```python
from build123d import *

# Parameters (mm, degrees)
SKETCH1_R                           = 1.5
BOSS_EXTRUDE1_DEPTH                 = 42
SKETCH2_R                           = 2.75
BOSS_EXTRUDE2_DEPTH                 = 2.2
ESCALA1_SCALE                       = 1.5
ESCALA2_SCALE                       = 1.5
CROQUIS1_R                          = 3.4
SALIENTE_EXTRUIR1_DEPTH             = 10
SALIENTE_EXTRUIR1_DIRECTION_2_REACH = 96.904


with BuildPart() as part:
    # Sketch1 → Boss-Extrude1 (new body)
    with BuildSketch(Plane.XY):
        with Locations(Location((0, 0, 0), (0, 0, 180))):
            Circle(SKETCH1_R)
    extrude(amount=BOSS_EXTRUDE1_DEPTH)

    # Sketch2 → Boss-Extrude2 (add)
    with BuildSketch(Plane(origin=(0, 0, 0), x_dir=(-1, 0, 0), z_dir=(0, 0, -1))):
        Circle(SKETCH2_R)
    extrude(amount=-BOSS_EXTRUDE2_DEPTH)


with BuildPart() as part_1:
    # Escala1: scaled about (0, 0, 0)
    add(part.part.scale(ESCALA1_SCALE))


with BuildPart() as part_2:
    # Escala2: scaled about (0, 0, 0)
    add(part_1.part.scale(ESCALA2_SCALE))

    # Croquis1 → Saliente-Extruir1 (add)
    with BuildSketch(Plane.XY.offset(94.5)):
        Circle(CROQUIS1_R)
    extrude(amount=SALIENTE_EXTRUIR1_DEPTH)

    # Croquis1 → Saliente-Extruir1 direction 2 (add, up to next)
    with BuildSketch(Plane.XY.offset(94.5), mode=Mode.PRIVATE) as saliente_extruir1_direction_2_sk1:
        Circle(CROQUIS1_R)
    saliente_extruir1_direction_2_tool1 = extrude(saliente_extruir1_direction_2_sk1.sketch, amount=-SALIENTE_EXTRUIR1_DIRECTION_2_REACH, mode=Mode.PRIVATE) - part_2.part
    add(saliente_extruir1_direction_2_tool1.solids().sort_by_distance((0, 0, 94.5))[0])


solid = part_2.part
```
Can you work these out from the model? Positions are in its coordinate system, mm. A direction names the side the tool comes from. Coordinates: 2 decimals unless noted, no trailing zeros. Loops run counter-clockwise (first coordinate to the right, second up) from the corner with the lowest first, then second, coordinate; pieces in that order, holes last.
1) For pin 1 (5 mm diameter, centred on y = -4, z = 39, fed in from +X); pin 2 (5 mm diameter, centred on x = 1.5, z = 45, fed in from +Y); pin 3 (4 mm diameter, centred on x = 3, z = 62, fed in from -Y), each with a flat end and sliding along its axis, tell me the tip position at first contact or that it passes through.
2) Imagine slicing it at D-D on y = -4.25. List the corners of the cut face in (x, z) for me.
3) I need wall thicknesses on probe 1 along Z at (x, y) = (1, -3.5); probe 2 along X at (y, z) = (-0.25, 13); probe 3 along X at (y, z) = (-1.5, 83.5). Which ranges of each line are inside material? Lowest first, please.
4) Imagine slicing it at A-A on x = 0. List the corners of the cut face in (y, z) for me, plus the area to 3 significant figures.
5) Imagine slicing it at C-C on z = 23. List the corners of the cut face in (x, y) for me, plus the area to 3 significant figures.
6) Which directions (+Z, -Z, +X, -X, +Y, -Y) give clear straight access to the entire face, cutting with the end or side of a thin tool? Please do faces 1 (the cylindrical face through (-0.74, -3.32, 55.42)), 2 (the flat face through (0, 0, 104.5)).
Completed:
1. pin 1: stops at x = 3.05
1. pin 2: stops at y = 3.4
1. pin 3: stops at y = -3.25
2. outline: (-4.5, 0) - (4.5, 0) - (4.5, 4.95) - (-4.5, 4.95) - close
3. probe 1: z = 0 to 4.95
3. probe 2: x = -3.39 to 3.39
3. probe 3: x = -3.05 to 3.05
4. outline: (-6.19, 0) - (6.19, 0) - (6.19, 4.95) - (3.4, 4.95) - (3.4, 104.5) - (-3.4, 104.5) - (-3.4, 4.95) - (-6.19, 4.95) - close
4. area: 738 mm2
5. outline: circle Ø6.8 at (0, 0)
5. area: 36.3 mm2
6. face 1: +Z
6. face 2: +Z, +X, -X, +Y, -Y
